from build123d import *

# Parameters (mm, degrees)
F1_DEPTH = 6.35


# Not quite as in the source:
# - ends of sketch curves that miss each other by under 0.0002 mm in the source are joined
# - the dataset's text gives a spline's control points without its knots; the knots are read off the source's solid


with BuildPart() as f1:
    # F0 (on Front) → F1 (new body, symmetric)
    with BuildSketch(Plane.XZ):
        with BuildLine():
            Line((-8.4141566916, -5.3975), (0, -5.3975))
            ThreePointArc((0, -5.3975), (0.4871232852, -5.375473668), (0.9702708263, -5.3095744437))
            ThreePointArc((0.9702708263, -5.3095744437), (4.4301700946, -5.3015138122), (1.778, -3.0795863359))
            ThreePointArc((1.778, -3.0795863359), (-1.7391660801, -3.101682986), (-3.5548772461, -0.0893519188))
            ThreePointArc((-3.5548772461, -0.0893519188), (-3.5177568499, 0.5201180106), (-3.3769182629, 1.1142526848))
            add(Edge.make_bspline(
                [(-3.3769182629, 1.1142526848), (-3.213886893, 2.2483634663), (-3.0651248799, 3.384623456), (-2.942596945, 4.524834745)],
                knots=[0.1529319216, 0.1529319216, 0.1529319216, 0.1529319216, 0.2811638974, 0.2811638974, 0.2811638974, 0.2811638974], degree=3))
            ThreePointArc((-2.942596945, 4.524834745), (-3.9835985246, 3.6419704892), (-4.7698383359, 2.5261924906))
            add(Edge.make_bspline(
                [(-5.3975, -1.7347033349), (-5.173779235, -0.3165887052), (-4.9567128934, 1.1025281941), (-4.7698383359, 2.5261924906)],
                knots=[0.0454256059, 0.0454256059, 0.0454256059, 0.0454256059, 0.2061005135, 0.2061005135, 0.2061005135, 0.2061005135], degree=3))
            Line((-5.3975, -1.7347033349), (-5.3975, -2.1827106738))
            ThreePointArc((-5.3975, -2.1827106738), (-5.4459433862, -2.5718905674), (-5.5883169948, -2.9373184082))
            ThreePointArc((-5.5883169948, -2.9373184082), (-6.1719143737, -3.5461797839), (-6.985, -3.7702106738))
            ThreePointArc((-6.985, -3.7702106738), (-7.7980896495, -3.5461803993), (-8.3816869181, -2.9373205224))
            add(Edge.make_bspline(
                [(-8.3816869181, -2.9373205224), (-7.6903162591, 1.4077055077), (-6.2862259108, 10.2319288559), (-7.676155344, 19.4769791983), (-8.3816869181, 24.1697893262)],
                knots=[0, 0, 0, 0, 0.4923975582, 1, 1, 1, 1], degree=3))
            ThreePointArc((-8.3816869181, 24.1697893262), (-6.985, 25.5664762444), (-5.5883130819, 24.1697893263))
            add(Edge.make_bspline(
                [(-4.676452861, 17.6339959576), (-4.9321460197, 19.8053249313), (-5.2602295508, 21.9875571288), (-5.5883130819, 24.1697893263)],
                knots=[0.7639566994, 0.7639566994, 0.7639566994, 0.7639566994, 1, 1, 1, 1], degree=3))
            ThreePointArc((-4.676452861, 17.6339959576), (-3.8112048513, 17.0315712658), (-3.1110035111, 17.8197893262))
            add(Edge.make_bspline(
                [(-3.1110035111, 17.8197893262), (-3.3633587069, 19.9297914909), (-3.6820858944, 22.0497904085), (-4.0008130819, 24.1697893262)],
                knots=[0.7706882235, 0.7706882235, 0.7706882235, 0.7706882235, 1, 1, 1, 1], degree=3))
            ThreePointArc((-4.0008130819, 24.1697893262), (-7.4285431353, 27.1208299985), (-9.837338265, 23.292556185))
            add(Edge.make_bspline(
                [(-9.8352581181, -3.3290753137), (-9.6597468246, -2.2260473952), (-9.3104483349, -0.0304942675), (-8.8571977057, 3.2414000554), (-8.5914867755, 5.9577245973), (-8.4768185316, 8.1311720824), (-8.4476359431, 9.7599621423), (-8.4814070197, 11.4021639111), (-8.5995564813, 13.6155987531), (-8.8666228021, 16.4200169888), (-9.3175498954, 19.8349473194), (-9.6635970859, 22.1369248922), (-9.837338265, 23.292556185)],
                knots=[0, 0, 0, 0, 0.125, 0.25, 0.375, 0.4375, 0.5, 0.5625, 0.625, 0.75, 0.875, 1, 1, 1, 1], degree=3))
            ThreePointArc((-9.8352581181, -3.3290753137), (-9.7481101941, -4.6955367779), (-8.5725, -5.3975))
            Line((-8.5725, -5.3975), (-8.4141566916, -5.3975))
        make_face()
        with BuildLine():
            ThreePointArc((-8.5725, -5.3975), (-8.4933283458, -5.399633381), (-8.4141566916, -5.3975))
            Line((-8.4141566916, -5.3975), (-8.5725, -5.3975))
        make_face()
        with BuildLine():
            add(Edge.make_bspline(
                [(-3.3769182629, 1.1142526848), (-3.213886893, 2.2483634663), (-3.0651248799, 3.384623456), (-2.942596945, 4.524834745)],
                knots=[0.1529319216, 0.1529319216, 0.1529319216, 0.1529319216, 0.2811638974, 0.2811638974, 0.2811638974, 0.2811638974], degree=3))
            ThreePointArc((-3.3769182629, 1.1142526848), (-1.2667947714, 3.3227047728), (1.778, 3.0795863359))
            ThreePointArc((1.778, 3.0795863359), (4.4301700946, 5.3015138122), (0.9702708263, 5.3095744437))
            ThreePointArc((0.9702708263, 5.3095744437), (-1.0613537009, 5.2921200451), (-2.942596945, 4.524834745))
        make_face()
        with BuildLine():
            add(Edge.make_bspline(
                [(-5.3975, -1.7347033349), (-5.173779235, -0.3165887052), (-4.9567128934, 1.1025281941), (-4.7698383359, 2.5261924906)],
                knots=[0.0454256059, 0.0454256059, 0.0454256059, 0.0454256059, 0.2061005135, 0.2061005135, 0.2061005135, 0.2061005135], degree=3))
            ThreePointArc((-4.7698383359, 2.5261924906), (-5.2382348491, 1.3014998717), (-5.3975, 0))
            Line((-5.3975, 0), (-5.3975, -1.7347033349))
        make_face()
    extrude(amount=F1_DEPTH, both=True)


solid = f1.part
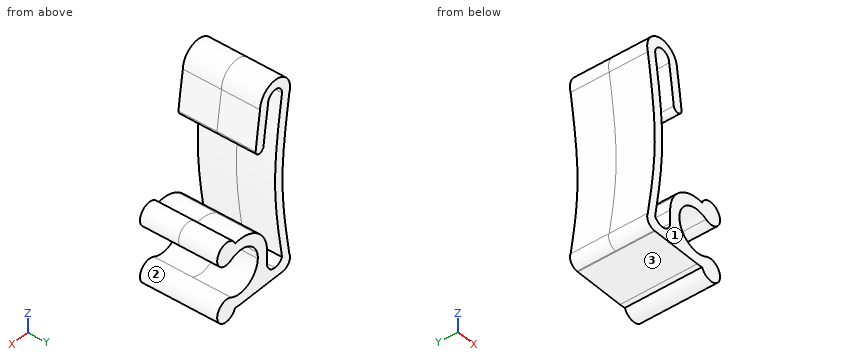
Can you work these out from the model? Positions are in its coordinate system, mm. Face numbers are marked on the shaded views. Coordinates: 2 decimals unless noted, no trailing zeros. Write each loop counter-clockwise with the first axis right and the second up, starting at its lowest first coordinate (ties: lowest second). Pieces come first, ordered by that corner, then holes. Notation, with made-up numbers: (-15.75, 1.5) -> (-5.75, 1.5) arc R17 ccw to (-5.75, 30.5) -> close; hole circle Ø1 at (83.25, -1). An arc over 180 degrees is marked (long way). Write each question's results on one line, items separated by ' | '. Start each with the question number.
Q1. I'm going to push flat-ended pins straight in: pin 1 (2.5 mm diameter, centred on y = -3, z = -1, fed in from -X); pin 2 (8 mm diameter, centred on x = -1, z = 19, fed in from +Y); pin 3 (4 mm diameter, centred on y = 3, z = 21, fed in from +X); pin 4 (2 mm diameter, centred on y = 0, z = -1, fed in from -X). Where does each tip first touch, or does it pass through?
Q2. Imagine slicing it at A-A (x = 3.5). Write out the boundary of the cut face in (y, z), then the cut area to 3 significant figures.
Q3. We'd pull the mould along Z, two halves only. Please class the marked faces 1, 2 and 3: +Z half, -Z half, draft (parallel to the pull), parting line (faces both ways), or undercut.
Q4. If I drill on probe 1 along Z at (x, y) = (0, 5); probe 2 along X at (y, z) = (-4.25, 18); probe 3 along Z at (x, y) = (-1, 2.5), over which ranges is the centre line in solid material (lowest first)?
Q5. Imagine slicing it at B-B (z = 25). Write out the boundary of the cut face in (x, y).
Taken from the geometry:
1) pin 1: stops at x = -9.66 | pin 2: stops at y = 6.35 | pin 3: stops at x = -3.26 | pin 4: stops at x = -9.62
2) outline: (-6.35, -6.33) -> (6.35, -6.33) -> (6.35, -3.02) -> (-6.35, -3.02) -> close; (-6.35, 3.02) -> (6.35, 3.02) -> (6.35, 6.33) -> (-6.35, 6.33) -> close | area: 84.2 mm^2
3) face 1: draft | face 2: undercut | face 3: -Z half
4) probe 1: z = -5.4 to -3.56, 3.56 to 5.4 | probe 2: x = -9.08 to -7.51, -4.72 to -3.13 | probe 3: z = -5.4 to -3.41, 3.41 to 5.3
5) outline: (-9.85, -6.35) -> (-8.11, -6.35) -> (-8.11, 6.35) -> (-9.85, 6.35) -> close; (-5.86, -6.35) -> (-4.12, -6.35) -> (-4.12, 6.35) -> (-5.86, 6.35) -> close
